from build123d import *

# Parameters (mm, degrees)
CROQUIS1_W                   = 13.84
CROQUIS1_H                   = 9.7
CROQUIS1_W_2                 = 1.1
CROQUIS1_H_2                 = 1.1
SALIENTE_EXTRUIR1_DEPTH      = 3
CROQUIS2_W                   = 13.84
CROQUIS2_H                   = 3
SALIENTE_EXTRUIR2_DEPTH      = 9.4
CORTAR_EXTRUIR1_DEPTH        = 16.490841585
SALIENTE_EXTRUIR3_DEPTH      = 13.5
SALIENTE_EXTRUIR3_DEPTH_BACK = 3.6
CROQUIS5_W                   = 1.1
CROQUIS5_H                   = 1.1


with BuildPart() as part:
    # Croquis1 → Saliente-Extruir1 (new body)
    with BuildSketch(Plane(origin=(0, 0, 0), x_dir=(1, 0, 0), z_dir=(0, 1, 0))):
        with Locations((5.08, 0.1)):
            Rectangle(CROQUIS1_W, CROQUIS1_H)
        Rectangle(CROQUIS1_W_2, CROQUIS1_H_2, mode=Mode.SUBTRACT)
        with Locations((10.16, 0)):
            Rectangle(CROQUIS1_W_2, CROQUIS1_H_2, mode=Mode.SUBTRACT)
        with Locations((5.08, 0)):
            Rectangle(CROQUIS1_W_2, CROQUIS1_H_2, mode=Mode.SUBTRACT)
    extrude(amount=SALIENTE_EXTRUIR1_DEPTH)

    # Croquis2 → Saliente-Extruir2 (add)
    with BuildSketch(Plane(origin=(0, 3, 0), x_dir=(1, 0, 0), z_dir=(0, 1, 0))):
        with Locations((5.08, 3.45)):
            Rectangle(CROQUIS2_W, CROQUIS2_H)
    extrude(amount=SALIENTE_EXTRUIR2_DEPTH)

    # Croquis3 → Cortar-Extruir1 (cut)
    with BuildSketch(Plane.ZY.offset(1.84)):
        with BuildLine():
            Line((-4.95, 12.4), (-4.95, 5.130923429))
            ThreePointArc((-4.95, 5.130923429), (-4.928460036, 5.292584893), (-4.865343077, 5.442966568))
            Line((-4.865343077, 5.442966568), (-3.238584298, 8.220392257))
            ThreePointArc((-3.238584298, 8.220392257), (-3.050389859, 8.882763545), (-3.206840185, 9.553342522))
            Line((-3.206840185, 9.553342522), (-4.429874218, 11.889875107))
            Line((-4.429874218, 11.889875107), (-3.455311447, 12.4))
            Line((-3.455311447, 12.4), (-4.95, 12.4))
        make_face()
        with BuildLine():
            Line((-1.95, 12.4), (-3.455311447, 12.4))
            Line((-3.455311447, 12.4), (-2.232277415, 10.063467416))
            ThreePointArc((-2.232277415, 10.063467416), (-2.021605007, 9.506586156), (-1.95, 8.9155089))
            Line((-1.95, 8.9155089), (-1.95, 12.4))
        make_face()
        with BuildLine():
            Line((-1.95, 3), (-1.95, 8.9155089))
            ThreePointArc((-1.95, 8.9155089), (-2.036358841, 8.267369623), (-2.28940975, 7.664453701))
            Line((-2.28940975, 7.664453701), (-3.85, 5))
            Line((-3.85, 5), (-3.85, 2.319959731))
            ThreePointArc((-3.85, 2.319959731), (-3.508458272, 1.760049187), (-2.854318236, 1.807497933))
            Line((-2.854318236, 1.807497933), (-1.184444515, 3))
            Line((-1.184444515, 3), (-1.95, 3))
        make_face()
    extrude(amount=-CORTAR_EXTRUIR1_DEPTH, mode=Mode.SUBTRACT)

    # Croquis5 → Saliente-Extruir3 (add, two sides: drawn at the far end of the back side and taken through both)
    with BuildSketch(Plane(origin=(0, 0, 0), x_dir=(1, 0, 0), z_dir=(0, 1, 0)).offset(-SALIENTE_EXTRUIR3_DEPTH_BACK)):
        with Locations((10.16, 0)):
            Rectangle(CROQUIS5_W, CROQUIS5_H)
        Rectangle(CROQUIS5_W, CROQUIS5_H)
        with Locations((5.08, 0)):
            Rectangle(CROQUIS5_W, CROQUIS5_H)
    extrude(amount=SALIENTE_EXTRUIR3_DEPTH + SALIENTE_EXTRUIR3_DEPTH_BACK)


solid = part.part
Work out the finished part from the listing and answer in its coordinate system (mm). A direction names the side the tool comes from. Coordinates: 2 decimals unless noted, no trailing zeros. Write each loop counter-clockwise with the first axis right and the second up, starting at its lowest first coordinate (ties: lowest second). Pieces come first, ordered by that corner, then holes. Notation, with made-up numbers: M -18,-30.75 L 14,-30.75 A29 cw 14,7.25 Z; hole C 73,59.5 d2. An arc over 180 degrees is marked long. Write item = value, one per line.
1. For faces 5 (the face through (0, -2, -0.55)), 6 (the face through (10.71, -2, 0)), 7 (the face through (0.55, 8, 0)), determine the directions among +Z, -Z, +X, -X, +Y, -Y from which every point of the face is accessible in a straight line to the end or side of a thin tool.
Solution:
face_5 = -Z, +X, -X, -Y
face_6 = +Z, -Z, +X, -Y
face_7 = +Z, +Y
2. The part is cut by section D-D (y = 4.5). Determine the outline of the cut face in (x, z), then the cut area to 3 significant figures.
Solution:
outline = M -1.84,-4.95 L 12,-4.95 L 12,-3.85 L -1.84,-3.85 Z; M -0.55,-0.55 L 0.55,-0.55 L 0.55,0.55 L -0.55,0.55 Z; M 4.53,-0.55 L 5.63,-0.55 L 5.63,0.55 L 4.53,0.55 Z; M 9.61,-0.55 L 10.71,-0.55 L 10.71,0.55 L 9.61,0.55 Z
area = 18.9 mm2
3. The part is cut by section A-A (y = -1.5). Determine the outline of the cut face in (x, z), then the cut area to 3 significant figures.
Solution:
outline = M -0.55,-0.55 L 0.55,-0.55 L 0.55,0.55 L -0.55,0.55 Z; M 4.53,-0.55 L 5.63,-0.55 L 5.63,0.55 L 4.53,0.55 Z; M 9.61,-0.55 L 10.71,-0.55 L 10.71,0.55 L 9.61,0.55 Z
area = 3.63 mm2
4. Straight lines are drawn through the part: line 1 (X direction, y = 6.25, z = -0.25); line 2 (Z direction, x = 1.25, y = 2.25); line 3 (Y direction, x = 11.75, z = -3.25). For each, find the intervals that lie inside material, in ascending order. Write a range as from..to.
Solution:
line_1 = -0.55..0.55, 4.53..5.63, 9.61..10.71
line_2 = -4.95..-3.85, -2.23..4.75
line_3 = 0..1.69, 6.02..8.2, 9.64..12.01
5. Determine the mould class of faces 1 (the face through (4.98, 8.87, -3.05)), 2 (the face through (0, -3.6, 0)), 3 (the face through (10.71, 8, 0)), 4 (the face through (10, 13.5, 0)) for opening direction Y: released by +Y, released by -Y, zero draft, split by the parting line, or undercut.
Solution:
face_1 = undercut
face_2 = released by -Y
face_3 = zero draft
face_4 = released by +Y
6. Flat-ended cylindrical pins translate along their axes: pin 1 (0.6 mm diameter, centred on y = -1.5, z = 0, fed in from -X); pin 2 (1.2 mm diameter, centred on x = 10, y = -1.5, fed in from +Z); pin 3 (1.2 mm diameter, centred on x = 5.5, y = 7.5, fed in from -Z). Find the tip coordinate at first contact, or state that the pin passes through.
Solution:
pin_1 = -0.55
pin_2 = 0.55
pin_3 = -4.01
7. The part is cut by section C-C (z = -2.5). Determine the outline of the cut face in (x, y), then the cut area to 3 significant figures.
Solution:
outline = M -1.84,0 L 12,0 L 12,2.06 L -1.84,2.06 Z; M -1.84,7.3 L 12,7.3 L 12,10.57 L -1.84,10.57 Z
area = 73.8 mm2
8. The part is cut by section B-B (x = 1.5). Determine the outline of the cut face in (y, z).
Solution:
outline = M 0,-4.95 L 5.13,-4.95 A0.62 ccw 5.44,-4.87 L 8.22,-3.24 A1.38 cw 9.55,-3.21 L 11.89,-4.43 L 12.4,-3.46 L 10.06,-2.23 A2.48 ccw 7.66,-2.29 L 5,-3.85 L 2.32,-3.85 A0.63 cw 1.81,-2.85 L 3,-1.18 L 3,4.75 L 0,4.75 Z
